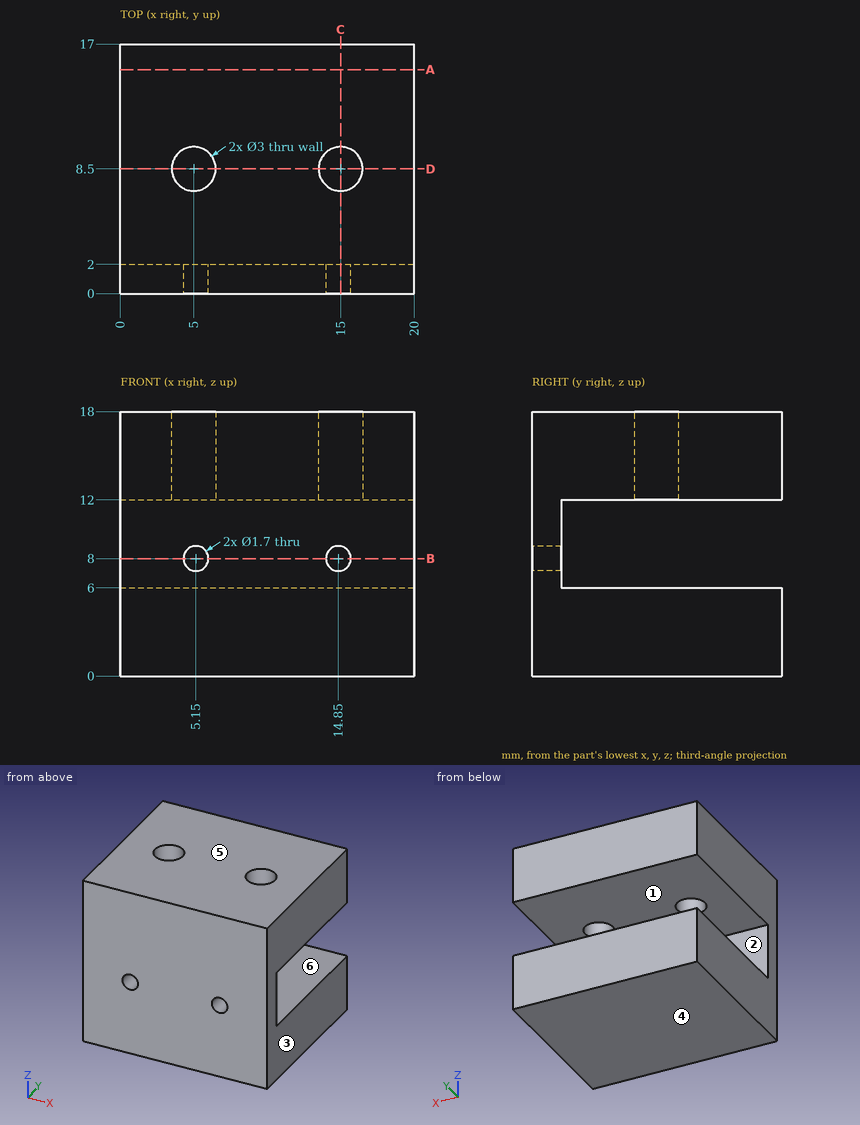
Part print with two shaded views. Sizes in mm from the minimum x, y, z corner. A direction names the side the tool comes from. Give positions to 0.01 mm unless a question says otherwise; leave off trailing zeros. Order: outer loops, then holes, each group sorted by start corner. A loop starts at its lowest first (then second) coordinate and runs counter-clockwise, first axis right, second up. Notation, with made-up numbers: M 9.25,3.5 L 23.25,3.5 A20 ccw 23.25,36.5 Z; hole C -9,-20.5 d8. An arc over 180 degrees is marked long. Write item = value, one per line.
Q1. Flat gauge pin, fed straight in: pin 1 (2.5 mm diameter, centred on x = 5, y = 8.5, fed in from +Z). Where does the tip first touch, or does it go through?
Derived:
pin_1 = 6
Q2. Drill centre lines: line 1 (Z direction, x = 14.5, y = 10.75); line 2 (Y direction, x = 15, z = 16.05); line 3 (Z direction, x = 14.85, y = 1.45). Where is each one in solid material? Low to high. Write a range as [from, to].
Derived:
line_1 = [0, 6], [12, 18]
line_2 = [0, 7], [10, 17]
line_3 = [0, 7.15], [8.85, 18]
Q3. Cut at A-A, the plane y = 15.25. List the corners of the cut face in (x, z).
Derived:
outline = M 0,0 L 20,0 L 20,6 L 0,6 Z; M 0,12 L 20,12 L 20,18 L 0,18 Z
Q4. Two-plate mould, pull along Z, no slides. Class the marked faces 1, 2, 3 and 4: pulls with the +Z half, pulls with the -Z half, needs draft (parallel to the pull), parting line crosses it, or undercut.
Derived:
face_1 = undercut
face_2 = undercut
face_3 = needs draft
face_4 = pulls with the -Z half
Q5. Cut at D-D, the plane y = 8.5. List the corners of the cut face in (x, z), then the cut area to 3 significant figures.
Derived:
outline = M 0,0 L 20,0 L 20,6 L 0,6 Z; M 0,12 L 3.5,12 L 3.5,18 L 0,18 Z; M 6.5,12 L 13.5,12 L 13.5,18 L 6.5,18 Z; M 16.5,12 L 20,12 L 20,18 L 16.5,18 Z
area = 204 mm2
Q6. Tool access for the marked faces 5 and 6: list every direction of +Z, -Z, +X, -X, +Y, -Y with a clear straight run to the whole face (end or side of a thin tool).
Derived:
face_5 = +Z, +X, -X, +Y, -Y
face_6 = +X, -X, +Y
Q7. Cut at C-C, the plane x = 15. List the corners of the cut face in (y, z), then the cut area to 3 significant figures.
Derived:
outline = M 0,0 L 17,0 L 17,6 L 2,6 L 2,7.16 L 0,7.16 Z; M 0,8.84 L 2,8.84 L 2,12 L 7,12 L 7,18 L 0,18 Z; M 10,12 L 17,12 L 17,18 L 10,18 Z
area = 195 mm2
Q8. Cut at B-B, the plane z = 8. List the corners of the cut face in (x, y).
Derived:
outline = M 0,0 L 4.3,0 L 4.3,2 L 0,2 Z; M 6,0 L 14,0 L 14,2 L 6,2 Z; M 15.7,0 L 20,0 L 20,2 L 15.7,2 Z
